Geometry: final body of the model. Coordinates: model frame, mm. A direction names the side the tool comes from. Coordinates: 2 decimals unless noted, no trailing zeros. Loops run counter-clockwise (first coordinate to the right, second up) from the corner with the lowest first, then second, coordinate; pieces in that order, holes last. Notation, with made-up numbers: (49.5, 15) -> (105.5, 15) arc R16 cw to (105.5, 32) -> close; hole circle Ø1 at (-39.5, 35.5). An arc over 180 degrees is marked (long way). One line per item, written item: value. Start each with the question number.
Item 1: Set-up query: faces 4 (the flat face through (-4.374, -0.07, 43.845)), 5 (the flat face through (-4, 0, 23)). Return all of +Z, -Z, +X, -X, +Y, -Y with unobstructed straight access to the full face (end or side cutting, diameter ignored); none if empty.
Item 2: Section query C-C on z = 16. Return loops of the section in (x, y).
Item 3: Section query A-A on y = 0.5. Return loops of the section in (x, z), then the cut area to 3 significant figures.
Item 4: Section query B-B on x = 0. Return loops of the section in (y, z), then the cut area to 3 significant figures.
Item 5: Mould query, pull axis X, two halves, no side actions, for faces 1 (the flat face through (-5, 0, 23)), 2 (the flat face through (0, -5, 24)), 3 (the flat face through (0, -4, 24)). Classes: +X half, -X half, draft (parallel to the pull), parting line (faces both ways), or undercut.
Item 6: Ray query, probe 1 along Y at (x, z) = (-0.5, 24.5); probe 2 along Y at (x, z) = (-3.5, 3). Return the intervals inside material, ascending. Write a range as from..to.
from build123d import *

# Parameters (mm, degrees)
SKETCH_1_W          = 10
SKETCH_1_H          = 10
SKETCH_1_W_2        = 8
SKETCH_1_H_2        = 8
EXTRUDE_1_DEPTH     = 200
FILLET_1_R          = 0.2
CUT_EXTRUDE_1_DEPTH = 201.31225624
CUT_EXTRUDE_2_DEPTH = 201.31225624


with BuildPart() as part:
    # 草圖1 → 填料-伸長1 (new body)
    with BuildSketch(Plane.XY):
        Rectangle(SKETCH_1_W, SKETCH_1_H)
        Rectangle(SKETCH_1_W_2, SKETCH_1_H_2, mode=Mode.SUBTRACT)
    extrude(amount=EXTRUDE_1_DEPTH)

    # 圓角1
    fillet_1_edges = [part.edges().sort_by_distance(p)[0] for p in [
        (-4, 4, 100),
        (-4, -4, 100),
        (4, -4, 100),
        (4, 4, 100),
        (-5, 5, 100),
        (5, 5, 100),
        (5, -5, 100),
        (-5, -5, 100),
    ]]
    fillet(fillet_1_edges, radius=FILLET_1_R)

    # 草圖2 → 除料-伸長1 (cut, through all)
    with BuildSketch(Plane(origin=(5, 0, 0), x_dir=(0, 0, -1), z_dir=(1, 0, 0))):
        Polygon((0, 5), (0, -5), (-3.639702343, -5), align=None)
    extrude(amount=-CUT_EXTRUDE_1_DEPTH, mode=Mode.SUBTRACT)

    # 草圖3 → 除料-伸長2 (cut, through all)
    with BuildSketch(Plane(origin=(5, 0, 0), x_dir=(0, 0, -1), z_dir=(1, 0, 0))):
        Polygon((-45.639702343, -5), (-42, 5), (-200, 5), (-200, -5), align=None)
    extrude(amount=-CUT_EXTRUDE_2_DEPTH, mode=Mode.SUBTRACT)


solid = part.part
Reply:
1. face 4: +Z, +X, -X, +Y
1. face 5: +Z, -Z
2. outline: (-5, -4.8) arc R0.2 ccw to (-4.8, -5) -> (4.8, -5) arc R0.2 ccw to (5, -4.8) -> (5, 4.8) arc R0.2 ccw to (4.8, 5) -> (-4.8, 5) arc R0.2 ccw to (-5, 4.8) -> close; hole (-4, -3.8) arc R0.2 ccw to (-3.8, -4) -> (3.8, -4) arc R0.2 ccw to (4, -3.8) -> (4, 3.8) arc R0.2 ccw to (3.8, 4) -> (-3.8, 4) arc R0.2 ccw to (-4, 3.8) -> close
3. outline: (-5, 1.64) -> (-4, 1.64) -> (-4, 43.64) -> (-5, 43.64) -> close; (4, 1.64) -> (5, 1.64) -> (5, 43.64) -> (4, 43.64) -> close
3. area: 84.0 mm²
4. outline: (-5, 3.64) -> (-4, 3.28) -> (-4, 45.28) -> (-5, 45.64) -> close; (4, 0.36) -> (5, 0) -> (5, 42) -> (4, 42.36) -> close
4. area: 84.0 mm²
5. face 1: -X half
5. face 2: draft
5. face 3: undercut
6. probe 1: y = -5..-4, 4..5
6. probe 2: y = 4..5
